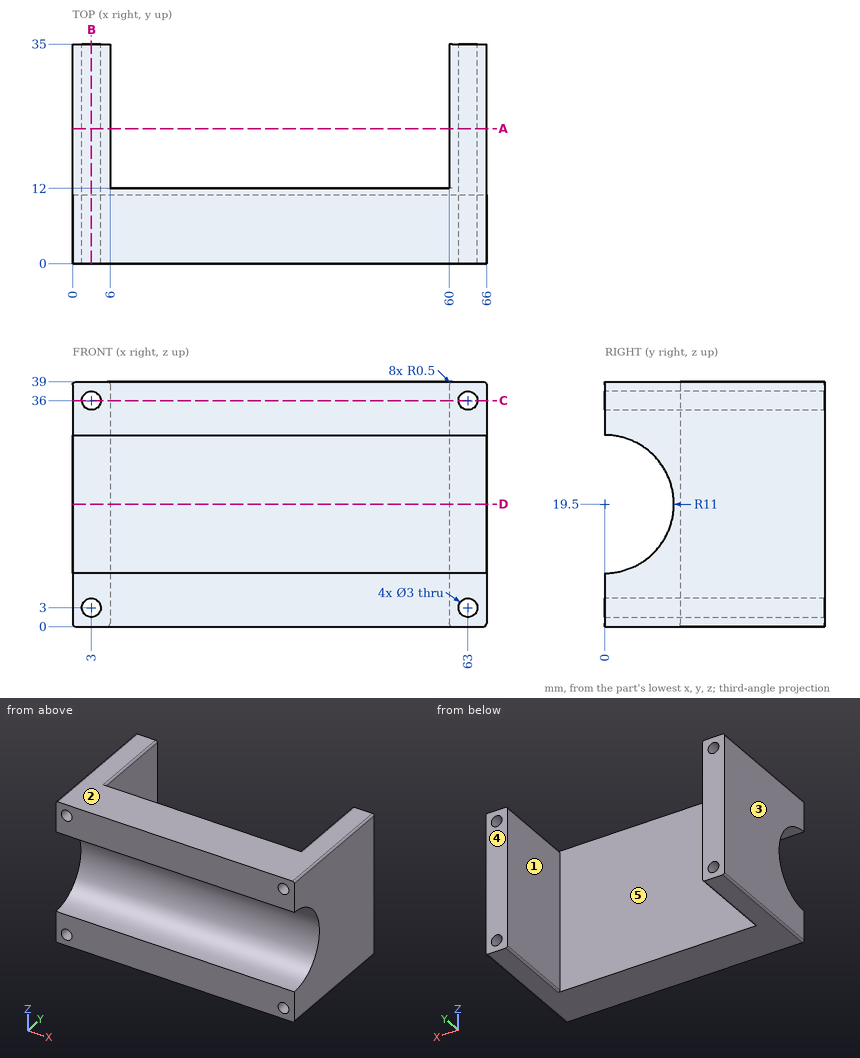
Answer from the drawing. Dimensions are ordinates in mm from the lowest x, y and z of the part. A direction names the side the tool comes from. Give positions to 0.01 mm unless a question says otherwise; leave off trailing zeros. Write each loop counter-clockwise with the first axis right and the second up, starting at its lowest first coordinate (ties: lowest second). Pieces come first, ordered by that corner, then holes.
1) Find the intervals of material crossed by L1, parallel to X at y = 21, z = 3; L2, parallel to X at y = 17, z = 33.5; L3, parallel to Z at x = 3.5, y = 4.5, in increasing order.
2) Section C-C (z = 36) is taken. Write down the section's boundary in (x, y).
3) Section A-A (y = 21.5) is taken. Write down the section's boundary in (x, z).
4) A tool of negligible diameter and unlimited length cuts with its end or side. For the marked faces 1 and 2, from which of +Z, -Z, +X, -X, +Y, -Y can it reach the whole face along a straight path? Write none if from no direction.
5) Given P1, Ø4, axis at x = 35.5, z = 23, coming from the +Y side; P2, Ø1, axis at x = 14.5, z = 27, coming from the -Y side, each flat-ended and moving along its own axis, determine where each tip first touches the part or whether it passes through.
6) Section B-B (x = 3) is taken. Write down the section's boundary in (y, z).
7) For a pull along X with two mould halves and no side action, classify the marked faces 3, 4 and 5 as pulls with the +X half, pulls with the -X half, needs draft (parallel to the pull), parting line crosses it, or undercut.
8) Section D-D (z = 19.5) is taken. Write down the section's boundary in (x, y).
Response:
1. L1: x = 0 to 1.5, 4.5 to 6, 60 to 61.5, 64.5 to 66
1. L2: x = 0 to 6, 60 to 66
1. L3: z = 0 to 1.59, 4.41 to 9.46, 29.54 to 34.59, 37.41 to 39
2. outline: (0, 0) - (1.5, 0) - (1.5, 35) - (0, 35) - close; (4.5, 0) - (61.5, 0) - (61.5, 35) - (60, 35) - (60, 12) - (6, 12) - (6, 35) - (4.5, 35) - close; (64.5, 0) - (66, 0) - (66, 35) - (64.5, 35) - close
3. outline: (0, 0.5) arc R0.5 ccw to (0.5, 0) - (5.5, 0) arc R0.5 ccw to (6, 0.5) - (6, 38.5) arc R0.5 ccw to (5.5, 39) - (0.5, 39) arc R0.5 ccw to (0, 38.5) - close; (60, 0.5) arc R0.5 ccw to (60.5, 0) - (65.5, 0) arc R0.5 ccw to (66, 0.5) - (66, 38.5) arc R0.5 ccw to (65.5, 39) - (60.5, 39) arc R0.5 ccw to (60, 38.5) - close; hole circle Ø3 at (3, 3); hole circle Ø3 at (3, 36); hole circle Ø3 at (63, 3); hole circle Ø3 at (63, 36)
4. face 1: +Z, -Z, +Y
4. face 2: +Z, +X, -X, +Y, -Y
5. P1: stops at y = 12
5. P2: stops at y = 7.55
6. outline: (0, 0) - (35, 0) - (35, 1.5) - (0, 1.5) - close; (0, 4.5) - (35, 4.5) - (35, 34.5) - (0, 34.5) - (0, 30.5) arc R11 cw to (0, 8.5) - close; (0, 37.5) - (35, 37.5) - (35, 39) - (0, 39) - close
7. face 3: pulls with the -X half
7. face 4: needs draft
7. face 5: undercut
8. outline: (0, 11) - (66, 11) - (66, 35) - (60, 35) - (60, 12) - (6, 12) - (6, 35) - (0, 35) - close
